For this review, take the finished solid that the model builds, in its own axes (mm). Give positions to 0.01 mm unless a question says otherwise; leave off trailing zeros. Order: outer loops, then holes, each group sorted by start corner. A loop starts at its lowest first (then second) coordinate and runs counter-clockwise, first axis right, second up. Notation, with made-up numbers: (12.5, 63) - (52.5, 63) arc R28 ccw to (52.5, 99) - close; hole circle Ø5 at (27.25, 22). An arc over 180 degrees is marked (long way). One line per item, written item: value.
```python
from build123d import *

# Parameters (mm, degrees)
SKETCH1_R           = 12.5
BOSS_EXTRUDE1_DEPTH = 1
SKETCH2_R           = 13.5
BOSS_EXTRUDE2_DEPTH = 1


with BuildPart() as part:
    # Sketch1 → Boss-Extrude1 (new body)
    with BuildSketch(Plane(origin=(0, 0, 0), x_dir=(1, 0, 0), z_dir=(0, 1, 0))):
        with BuildLine():
            Line((-7.795, 20.037164844), (-7.795, 25.157164844))
            Line((-7.795, 25.157164844), (7.795, 25.157164844))
            Line((7.795, 25.157164844), (7.795, 20.037164844))
            ThreePointArc((7.795, 20.037164844), (0, -21.5), (-7.795, 20.037164844))
        make_face()
        Circle(SKETCH1_R, mode=Mode.SUBTRACT)
    extrude(amount=BOSS_EXTRUDE1_DEPTH)

    # Sketch2 → Boss-Extrude2 (add)
    with BuildSketch(Plane.XZ):
        with BuildLine():
            Line((-6.795, -24.157164844), (6.795, -24.157164844))
            Line((6.795, -24.157164844), (6.795, -19.341095496))
            ThreePointArc((6.795, -19.341095496), (0, 20.5), (-6.795, -19.341095496))
            Line((-6.795, -19.341095496), (-6.795, -24.157164844))
        make_face()
        Circle(SKETCH2_R, mode=Mode.SUBTRACT)
    extrude(amount=BOSS_EXTRUDE2_DEPTH)


solid = part.part
```
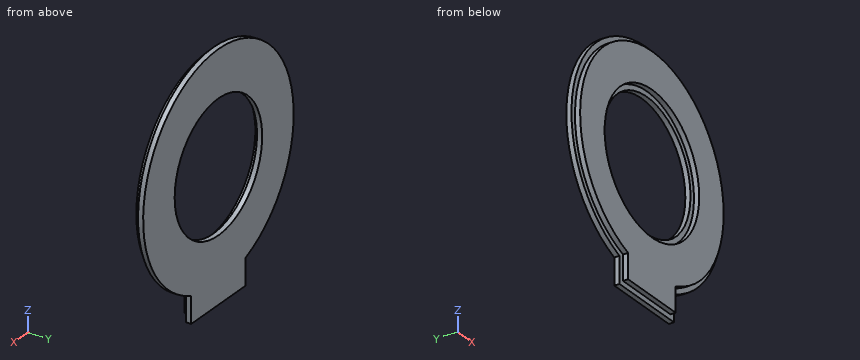
(1) Take a section at B-B (x = 0). Write out the cut boundary in (y, z), then the cut area to 3 significant figures.
Answers below:
outline: (-1, -24.16) - (0, -24.16) - (0, -25.16) - (1, -25.16) - (1, -12.5) - (0, -12.5) - (0, -13.5) - (-1, -13.5) - close; (-1, 13.5) - (0, 13.5) - (0, 12.5) - (1, 12.5) - (1, 21.5) - (0, 21.5) - (0, 20.5) - (-1, 20.5) - close
area: 39.3 mm^2
(2) Wall thickness on line 1 (Z direction, x = 0, y = 0.3); line 2 (X direction, y = 0.8, z = 0); line 3 (Z direction, x = 0, y = -0.65): over which ranges is each line inside the solid? List them lowest first. Write a range as from..to.
Answers below:
line 1: z = -25.16..-12.5, 12.5..21.5
line 2: x = -21.5..-12.5, 12.5..21.5
line 3: z = -24.16..-13.5, 13.5..20.5
(3) Take a section at A-A (z = 0). Write out the cut boundary in (x, y), then the cut area to 3 significant figures.
Answers below:
outline: (-21.5, 0) - (-20.5, 0) - (-20.5, -1) - (-13.5, -1) - (-13.5, 0) - (-12.5, 0) - (-12.5, 1) - (-21.5, 1) - close; (12.5, 0) - (13.5, 0) - (13.5, -1) - (20.5, -1) - (20.5, 0) - (21.5, 0) - (21.5, 1) - (12.5, 1) - close
area: 32.0 mm^2
(4) For P1, Ø0.8, axis at y = -0.5, z = -22.5, coming from the -X side (3 decimals); P2, Ø0.8, axis at y = -0.5, z = -21.5, coming from the +X side (3 decimals); P3, Ø1.1, axis at y = 0.5, z = -23, coming from the +X side (3 decimals), all flat-tipped, find the tip position at first contact; note any pin that passes through.
Answers below:
P1: stops at x = -6.795
P2: stops at x = 6.795
P3: stops at x = 7.795
(5) Take a section at C-C (y = 0.3). Write out the cut boundary in (x, z) (3 decimals), then the cut area to 3 significant figures.
Answers below:
outline: (-7.795, -25.157) - (7.795, -25.157) - (7.795, -20.037) arc R21.5 ccw (long way) to (-7.795, -20.037) - close; hole circle Ø25 at (0, 0)
area: 1,030 mm^2
(6) Take a section at D-D (z = -15). Write out the cut boundary in (x, y), then the cut area to 3 significant figures.
Answers below:
outline: (-15.4, 0) - (-13.97, 0) - (-13.97, -1) - (13.97, -1) - (13.97, 0) - (15.4, 0) - (15.4, 1) - (-15.4, 1) - close
area: 58.8 mm^2
